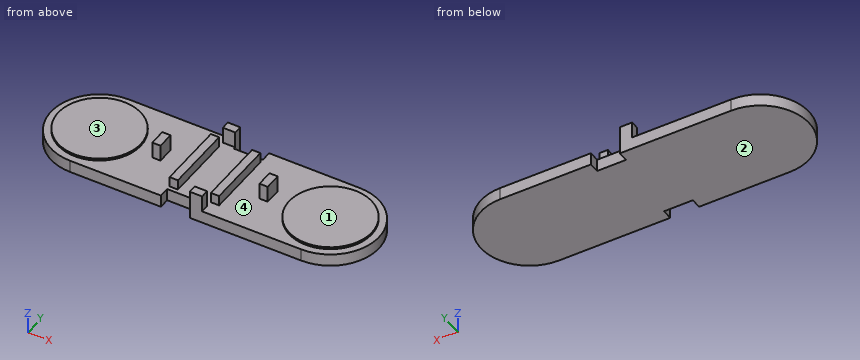
from build123d import *

# Parameters (mm, degrees)
PAD_DEPTH     = 3
SKETCH001_W   = 2
SKETCH001_H   = 16.5
PAD001_DEPTH  = 2.5
SKETCH002_W   = 2
SKETCH002_H   = 4
SKETCH002_W_2 = 3
SKETCH002_H_2 = 2
PAD002_DEPTH  = 4
SKETCH003_R   = 10
PAD003_DEPTH  = 0.5


with BuildPart() as part:
    # Sketch → Pad (new body)
    with BuildSketch(Plane.XY):
        with BuildLine():
            Line((-6, -9.25), (1, -9.25))
            Line((1, -11.75), (1, -9.25))
            Line((1, -11.75), (27.999978, -11.75))
            ThreePointArc((27.999978, -11.75), (39.749978, -1.2e-05), (28.000001, 11.75))
            Line((6, 11.75), (28.000001, 11.75))
            Line((6, 9.25), (6, 11.75))
            Line((6, 9.25), (-1, 9.25))
            Line((-1, 9.25), (-1, 11.75))
            Line((-1, 11.75), (-27.999999, 11.75))
            ThreePointArc((-27.999999, 11.75), (-39.749976, 1e-06), (-28.000001, -11.75))
            Line((-6, -11.75), (-28.000001, -11.75))
            Line((-6, -9.25), (-6, -11.75))
        make_face()
    extrude(amount=PAD_DEPTH)

    # Sketch001 (on Face14 of Pad) → Pad001 (join)
    with BuildSketch(Plane.XY.offset(3)):
        with Locations((-5, 0)):
            Rectangle(SKETCH001_W, SKETCH001_H)
        with Locations((5, 0)):
            Rectangle(SKETCH001_W, SKETCH001_H)
    extrude(amount=PAD001_DEPTH)

    # Sketch002 (on Face5 of Pad001) → Pad002 (join)
    with BuildSketch(Plane.XY.offset(3)):
        with Locations((-13, 0)):
            Rectangle(SKETCH002_W, SKETCH002_H)
        with Locations((13, 0)):
            Rectangle(SKETCH002_W, SKETCH002_H)
        with Locations((-2.5, 10.75)):
            Rectangle(SKETCH002_W_2, SKETCH002_H_2)
        with Locations((2.5, -10.75)):
            Rectangle(SKETCH002_W_2, SKETCH002_H_2)
    extrude(amount=PAD002_DEPTH)

    # Sketch003 (on Face5 of Pad002) → Pad003 (join)
    with BuildSketch(Plane.XY.offset(3)):
        with Locations((-28, 0)):
            Circle(SKETCH003_R)
        with Locations((28, 0)):
            Circle(SKETCH003_R)
    extrude(amount=PAD003_DEPTH)


solid = part.part
The listing builds one solid part. Answer for the finished solid, in the listing's coordinates (mm). Face numbers are marked on the shaded views. A direction names the side the tool comes from. Round coordinates to 2 decimals unless told otherwise and drop trailing zeros. Order: outer loops, then holes, each group sorted by start corner. A loop starts at its lowest first (then second) coordinate and runs counter-clockwise, first axis right, second up. Notation, with made-up numbers: (-6.5, 69.5) -> (21.5, 69.5) arc R16 cw to (21.5, 85.5) -> close; hole circle Ø8 at (7.5, 13). An arc over 180 degrees is marked (long way). Write each question's results on one line, items separated by ' | '. Start each with the question number.
Q1. Find section B-B (y = 0). Determine the outline of the cut face in (x, z).
Q2. The mould has two halves that part along X. Classify the marked faces 3 and 4: pulls with the +X half, pulls with the -X half, needs draft (parallel to the pull), parting line crosses it, or undercut.
Q3. Find section C-C (x = 13). Determine the outline of the cut face in (y, z).
Q4. Find section D-D (y = 4). Determine the outline of the cut face in (x, z).
Q5. Which of the six approach directions +Z, -Z, +X, -X, +Y, -Y give full straight-line access (tool end or side, diameter ignored) to the marked faces 1 and 2?
Q6. Each of these flat-tipped pins is pushed along its axis until it touches: pin 1 (1.6 mm diameter, centred on y = -11, z = 4.5, fed in from +X); pin 2 (1 mm diameter, centred on y = 2.5, z = 2, fed in from +X); pin 3 (12 mm diameter, centred on x = 0.5, y = 2, fed in from +Z); pin 4 (3 mm diameter, centred on x = -10, y = -5, fed in from -Z). Where does it stop, or does it pass through?
Q7. Straight lines are drawn through the part: probe 1 along X at (y, z) = (1.25, 6); probe 2 along X at (y, z) = (6.5, 4); probe 3 along Y at (x, z) = (-12.5, 6.25). For each, find the intervals that lie inside material, in ascending order. Write a range as from..to.
Q8. Find section A-A (x = 3). Determine the outline of the cut face in (y, z), then the cut area to 3 significant figures.
Worked answers:
1) outline: (-39.75, 0) -> (39.75, 0) -> (39.75, 3) -> (38, 3) -> (38, 3.5) -> (18, 3.5) -> (18, 3) -> (14, 3) -> (14, 7) -> (12, 7) -> (12, 3) -> (6, 3) -> (6, 5.5) -> (4, 5.5) -> (4, 3) -> (-4, 3) -> (-4, 5.5) -> (-6, 5.5) -> (-6, 3) -> (-12, 3) -> (-12, 7) -> (-14, 7) -> (-14, 3) -> (-18, 3) -> (-18, 3.5) -> (-38, 3.5) -> (-38, 3) -> (-39.75, 3) -> close
2) face 3: needs draft | face 4: undercut
3) outline: (-11.75, 0) -> (11.75, 0) -> (11.75, 3) -> (2, 3) -> (2, 7) -> (-2, 7) -> (-2, 3) -> (-11.75, 3) -> close
4) outline: (-39.05, 0) -> (39.05, 0) -> (39.05, 3) -> (37.17, 3) -> (37.17, 3.5) -> (18.83, 3.5) -> (18.83, 3) -> (6, 3) -> (6, 5.5) -> (4, 5.5) -> (4, 3) -> (-4, 3) -> (-4, 5.5) -> (-6, 5.5) -> (-6, 3) -> (-18.83, 3) -> (-18.83, 3.5) -> (-37.17, 3.5) -> (-37.17, 3) -> (-39.05, 3) -> close
5) face 1: +Z, +X, +Y, -Y | face 2: -Z, +X, -X, +Y, -Y
6) pin 1: stops at x = 4 | pin 2: stops at x = 39.58 | pin 3: stops at z = 5.5 | pin 4: stops at z = 0
7) probe 1: x = -14..-12, 12..14 | probe 2: x = -6..-4, 4..6 | probe 3: y = -2..2
8) outline: (-11.75, 0) -> (9.25, 0) -> (9.25, 3) -> (-9.75, 3) -> (-9.75, 7) -> (-11.75, 7) -> close | area: 71.0 mm2
